Check sheet for the modelled part. Datum: model origin and axes. Units: mm. A direction names the side the tool comes from. Give positions to 0.01 mm unless a question says otherwise; leave off trailing zeros. Write each loop counter-clockwise with the first axis right and the second up, starting at its lowest first coordinate (ties: lowest second). Pieces come first, ordered by that corner, then holes.
from build123d import *

# Parameters (mm, degrees)
ESQUISSE1_W             = 70
ESQUISSE1_H             = 67
ESQUISSE1_W_2           = 53.28358209
ESQUISSE1_H_2           = 51
BOSS_EXTRU_1_DEPTH      = 10
ESQUISSE2_W             = 8.358208955
ESQUISSE2_H             = 51
ENL_V_MAT_EXTRU_1_DEPTH = 5
ESQUISSE3_W             = 4
ESQUISSE3_H             = 4
ENL_V_MAT_EXTRU_2_DEPTH = 68
ENL_V_MAT_EXTRU_3_DEPTH = 5


with BuildPart() as part:
    # Esquisse1 → Boss.-Extru.1 (new body)
    with BuildSketch(Plane(origin=(0, 0, 0), x_dir=(1, 0, 0), z_dir=(0, 1, 0))):
        Rectangle(ESQUISSE1_W, ESQUISSE1_H)
        Rectangle(ESQUISSE1_W_2, ESQUISSE1_H_2, mode=Mode.SUBTRACT)
    extrude(amount=BOSS_EXTRU_1_DEPTH)

    # Esquisse2 → Enlèv. mat.-Extru.1 (cut)
    with BuildSketch(Plane(origin=(0, 10, 0), x_dir=(1, 0, 0), z_dir=(0, 1, 0))):
        with Locations((-30.820895523, 0)):
            Rectangle(ESQUISSE2_W, ESQUISSE2_H)
        with Locations((30.820895523, 0)):
            Rectangle(ESQUISSE2_W, ESQUISSE2_H)
    extrude(amount=-ENL_V_MAT_EXTRU_1_DEPTH, mode=Mode.SUBTRACT)

    # Esquisse3 → Enlèv. mat.-Extru.2 (cut, through all)
    with BuildSketch(Plane.XY.offset(33.5)):
        with Locations((33, 5)):
            Rectangle(ESQUISSE3_W, ESQUISSE3_H)
        with Locations((-33, 5)):
            Rectangle(ESQUISSE3_W, ESQUISSE3_H)
    extrude(amount=-ENL_V_MAT_EXTRU_2_DEPTH, mode=Mode.SUBTRACT)

    # Esquisse4 → Enlèv. mat.-Extru.3 (cut)
    with BuildSketch(Plane(origin=(0, 10, 0), x_dir=(1, 0, 0), z_dir=(0, 1, 0))):
        with BuildLine():
            Line((-28, 29.5), (28, 29.5))
            ThreePointArc((28, 29.5), (29, 28.5), (28, 27.5))
            Line((28, 27.5), (-28, 27.5))
            ThreePointArc((-28, 27.5), (-29, 28.5), (-28, 29.5))
        make_face()
        with BuildLine():
            Line((28, -30), (-28, -30))
            ThreePointArc((-28, -30), (-29, -29), (-28, -28))
            Line((-28, -28), (28, -28))
            ThreePointArc((28, -28), (29, -29), (28, -30))
        make_face()
    extrude(amount=-ENL_V_MAT_EXTRU_3_DEPTH, mode=Mode.SUBTRACT)


solid = part.part
1) Sectioned sample at B-B on x = -13. Record the boundary of the cut face in (y, z), then the cut area to 3 significant figures.
2) Access from +Z, -Z, +X, -X, +Y, -Y to the whole of each face (thin tool, end or side, straight path). Record for faces 1 (the flat face through (0, 8, -27.5)), 2 (the flat face through (-29, 5, 0)), 3 (the flat face through (33, 3, 0)), 4 (the flat face through (0, 5, 33.5)), 5 (the flat face through (-33, 7, -29)).
3) Draft check along Y on faces 6 (the flat face through (0, 5, -29)), 7 (the flat face through (35, 8, -29)), 8 (the flat face through (33, 7, 30)). Enter one of: +Y half, -Y half, draft (parallel to the pull), parting line (faces both ways), or undercut.
4) Sectioned sample at C-C on z = 10. Record the boundary of the cut face in (x, y), then the cut area to 3 significant figures.
5) Scan lines: L1, parallel to Z at x = -17.5, y = 7; L2, parallel to X at y = 2.25, z = -7.5; L3, parallel to Z at x = 18.5, y = 4.75. Record each from-to range of solid material in increasing order.
6) Sectioned sample at A-A on y = 8.5. Record the boundary of the cut face in (x, z).
7) Sectioned sample at D-D on x = 30. Record the boundary of the cut face in (y, z).
8) Gauge pin test, flat ends, axial feed: pin 1 (3 mm diameter, centred on y = 6, z = 12.5, fed in from +X); pin 2 (12 mm diameter, centred on x = -18, z = -1.5, fed in from +Y); pin 3 (2 mm diameter, centred on x = -33, z = -10, fed in from +Y); pin 4 (4.5 mm diameter, centred on x = 32.5, z = -8, fed in from +Y). Record the tip position at first contact, or that the pin passes through.
Answers below:
1. outline: (0, -33.5) - (10, -33.5) - (10, -29.5) - (5, -29.5) - (5, -27.5) - (10, -27.5) - (10, -25.5) - (0, -25.5) - close; (0, 25.5) - (10, 25.5) - (10, 28) - (5, 28) - (5, 30) - (10, 30) - (10, 33.5) - (0, 33.5) - close
1. area: 140 mm2
2. face 1: +Y
2. face 2: +X, -X, +Y
2. face 3: +Z, -Z, +X
2. face 4: +Z, +X, -X, +Y, -Y
2. face 5: +Z, -Z, -X
3. face 6: +Y half
3. face 7: draft
3. face 8: undercut
4. outline: (-35, 0) - (-26.64, 0) - (-26.64, 5) - (-31, 5) - (-31, 3) - (-35, 3) - close; (26.64, 0) - (35, 0) - (35, 3) - (31, 3) - (31, 5) - (26.64, 5) - close
4. area: 67.6 mm2
5. L1: z = -33.5 to -29.5, -27.5 to -25.5, 25.5 to 28, 30 to 33.5
5. L2: x = -35 to -26.64, 26.64 to 35
5. L3: z = -33.5 to -25.5, 25.5 to 33.5
6. outline: (-35, -33.5) - (35, -33.5) - (35, -25.5) - (-35, -25.5) - close; (-35, 25.5) - (35, 25.5) - (35, 33.5) - (-35, 33.5) - close; hole (-28, -29.5) - (28, -29.5) arc R1 ccw to (28, -27.5) - (-28, -27.5) arc R1 ccw to start; hole (-28, 28) - (28, 28) arc R1 ccw to (28, 30) - (-28, 30) arc R1 ccw to start
7. outline: (0, -33.5) - (10, -33.5) - (10, -25.5) - (5, -25.5) - (5, 25.5) - (10, 25.5) - (10, 33.5) - (0, 33.5) - close
8. pin 1: stops at x = 31
8. pin 2: passes through
8. pin 3: stops at y = 3
8. pin 4: stops at y = 5
